from build123d import *

# Parameters (mm, degrees)
F0_R     = 8.25
F0_W     = 10.5
F0_H     = 2.6
F1_DEPTH = 3
F0_H_2   = 14.9
F2_DEPTH = 5.7
F3_DEPTH = 13.5


with BuildPart() as f1:
    # F0 (on Front) → F1 (new body)
    with BuildSketch(Plane.XZ):
        Polygon((22.5, -10.25), (22.5, 10.25), (-22.5, 10.25), (-22.5, -10.25), (-5.25, -10.25), (-5.25, -7.65), (5.25, -7.65), (5.25, -10.25), align=None)
        with Locations((-13.1, 0)):
            Circle(F0_R, mode=Mode.SUBTRACT)
        with Locations((12.25, 0.25)):
            Circle(F0_R, mode=Mode.SUBTRACT)
        with Locations((0, -8.95)):
            Rectangle(F0_W, F0_H)
        with Locations((-13.1, 0)):
            Circle(F0_R)
        with Locations((12.25, 0.25)):
            Circle(F0_R)
    extrude(amount=F1_DEPTH)

    # F0 (on Front) → F2 (join)
    with BuildSketch(Plane.XZ):
        with Locations((0, -8.95)):
            Rectangle(F0_W, F0_H)
        with Locations((0, -17.7)):
            Rectangle(F0_W, F0_H_2)
    extrude(amount=-F2_DEPTH)

    # F0 (on Front) → F3 (join)
    with BuildSketch(Plane.XZ):
        with Locations((-13.1, 0)):
            Circle(F0_R)
        with Locations((12.25, 0.25)):
            Circle(F0_R)
    extrude(amount=F3_DEPTH)


solid = f1.part
The model under review builds one solid part; all positions refer to its coordinate system, in mm. A direction names the side the tool comes from. Coordinates: 2 decimals unless noted, no trailing zeros. Loops run counter-clockwise (first coordinate to the right, second up) from the corner with the lowest first, then second, coordinate; pieces in that order, holes last. Notation, with made-up numbers: M -35,82.25 L -22,82.25 A26 ccw -22,109.25 Z; hole C 65.5,70.25 d1. An arc over 180 degrees is marked long. Put each result on its own line as item: value. Start each with the question number.
Q1. Add section B-B (y = -5.75). Write out the cut boundary in (x, z).
Q2. Add section C-C (z = -3). Write out the cut boundary in (x, y), and give its area (3 significant figures).
Q3. The part is to be moulded in two halves that separate along X. For faces 4 (the flat face through (0, -3, 0)), 5 (the flat face through (0, 3, -7.65)), 6 (the flat face through (22.5, -1, 0)), say which applies: +X half, -X half, draft (parallel to the pull), parting line (faces both ways), or undercut.
Q4. For faces 1 (the flat face through (-22.5, -1, 0)), 2 (the flat face through (0, 0, -18)), 3 (the cylindrical face through (-5.23, -8.18, 2.48)), list the 3-axis set-ups (+Z, -Z, +X, -X, +Y, -Y) from which the entire face can be reached by the end or side of a thin tool; tool diameter is ignored.
Q5. Add section D-D (y = -2). Write out the cut boundary in (x, z).
Q6. Clearance check with flat-ended pins moving along their axes: pin 1 (1.5 mm diameter, centred on x = 16.5, y = -9, fed in from +Z); pin 2 (2.5 mm diameter, centred on x = -1, y = -2, fed in from -Z); pin 3 (11.5 mm diameter, centred on x = 0.5, z = -14, fed in from -Y); pin 4 (4 mm diameter, centred on x = 16, y = -4.5, fed in from +Z). State where each tip first meets the part, or that it passes through.
Q7. Add section A-A (x = 1). Write out the cut boundary in (y, z), and give its area (3 significant figures).
Q8. Wall thickness on line 1 (X direction, y = 1.25, z = -19.5); line 2 (Y direction, x = 0, z = 7.5); line 3 (Z direction, x = -2.5, y = 4.5): over which ranges is each line inside the solid? List them lowest first.
Answers:
1. outline: C -13.1,0 d16.5; C 12.25,0.25 d16.5
2. outline: M -22.5,-3 L -20.79,-3 L -20.79,-13.5 L -5.41,-13.5 L -5.41,-3 L 4.67,-3 L 4.67,-13.5 L 19.83,-13.5 L 19.83,-3 L 22.5,-3 L 22.5,0 L -22.5,0 Z
2. area: 456 mm^2
3. face 4: undercut
3. face 5: draft
3. face 6: +X half
4. face 1: +Z, -Z, -X, +Y, -Y
4. face 2: -Z, +X, -X, -Y
4. face 3: -Y
5. outline: M -22.5,-10.25 L 22.5,-10.25 L 22.5,10.25 L -22.5,10.25 Z
6. pin 1: stops at z = 7.72
6. pin 2: stops at z = -10.25
6. pin 3: stops at y = -3
6. pin 4: stops at z = 10.25
7. outline: M -3,-10.25 L 0,-10.25 L 0,-25.15 L 5.7,-25.15 L 5.7,-7.65 L 0,-7.65 L 0,10.25 L -3,10.25 Z
7. area: 161 mm^2
8. line 1: x = -5.25 to 5.25
8. line 2: y = -3 to 0
8. line 3: z = -25.15 to -7.65
